Could you check a few things on this model? Use its own coordinates, in mm. A direction names the side the tool comes from. Coordinates: 2 decimals unless noted, no trailing zeros. Write each loop counter-clockwise with the first axis right and the second up, starting at its lowest first coordinate (ties: lowest second). Pieces come first, ordered by that corner, then holes. Notation, with made-up numbers: M -14.5,76.5 L 34.5,76.5 A26 cw 34.5,98.5 Z; hole C -29,23 d10. An arc over 180 degrees is marked long. Write item = value, one per line.
```python
from build123d import *

# Parameters (mm, degrees)
F1_DEPTH  = 25.4
F3_DEPTH  = 12.7
F5_DEPTH  = 12.7
F7_DEPTH  = 12.7
F9_DEPTH  = 12.7
F10_DEPTH = 12.7


with BuildPart() as f1:
    # F0 (on Top) → F1 (new body)
    with BuildSketch(Plane.XY):
        with BuildLine():
            ThreePointArc((0, 6.35), (1.8598719395, 1.8598719395), (6.35, 0))
            Line((6.35, 0), (69.85, 0))
            ThreePointArc((69.85, 0), (74.3401280605, 1.8598719395), (76.2, 6.35))
            Line((76.2, 6.35), (76.2, 12.7))
            Line((76.2, 12.7), (63.5, 12.7))
            Line((63.5, 12.7), (63.5, 25.4))
            Line((63.5, 25.4), (63.5, 38.1))
            Line((63.5, 38.1), (76.2, 38.1))
            Line((76.2, 38.1), (76.2, 44.45))
            ThreePointArc((76.2, 44.45), (74.3401280605, 48.9401280605), (69.85, 50.8))
            Line((69.85, 50.8), (6.35, 50.8))
            ThreePointArc((6.35, 50.8), (1.8598719395, 48.9401280605), (0, 44.45))
            Line((0, 44.45), (0, 38.1))
            Line((0, 38.1), (12.7, 38.1))
            Line((12.7, 38.1), (12.7, 25.4))
            Line((12.7, 25.4), (12.7, 12.7))
            Line((12.7, 12.7), (0, 12.7))
            Line((0, 12.7), (0, 6.35))
        make_face()
    extrude(amount=F1_DEPTH)

    # F2 (on face) → F3 (join)
    with BuildSketch(Plane(origin=(0, 0, 0), x_dir=(1, 0, 0), z_dir=(0, 0, -1))):
        Polygon((63.5, -12.7), (63.5, 0), (50.8120395243, 0), (50.8120395243, -50.8), (63.5, -50.8), (63.5, -38.1), align=None)
        Polygon((25.4, -50.8), (25.4, 0), (12.7, 0), (12.7, -12.7), (12.7, -38.1), (12.7, -50.8), align=None)
    extrude(amount=F3_DEPTH)

    # F4 (on face) → F5 (join)
    with BuildSketch(Plane.XY.offset(25.4)):
        Polygon((19.5285081863, 50.8), (38.1, 0), (53.2767996192, 50.8), align=None)
    extrude(amount=F5_DEPTH)

    # F6 (on face) → F7 (join)
    with BuildSketch(Plane.XY.offset(38.1)):
        Polygon((19.5285081863, 50.8), (28.8142540932, 25.4), (45.6883998096, 25.4), (53.2767996192, 50.8), align=None)
    extrude(amount=F7_DEPTH)

    # F10 (add): a face of the model
    f10_faces = [f1.faces().sort_by_distance(p)[0] for p in [
        (36.7798419244, 39.5111111111, 50.8),
    ]]


with BuildPart() as f9:
    # F8 (on face) → F9 (new body)
    with BuildSketch(Plane.XY.offset(50.8)):
        Polygon((45.6883998096, 25.4), (28.8142540932, 25.4), (37.9194319248, 0), align=None)
    extrude(amount=F9_DEPTH)


with BuildPart() as f1_1:
    add(f1.part)

    add(f9.part)  # F10 merges F9
    extrude(f10_faces, amount=F10_DEPTH)


solid = f1_1.part
```
Item 1: I'm going to push flat-ended pins straight in: P1, Ø4, axis at x = 30, y = 34.5, coming from the -Z side; P2, Ø4, axis at x = 36.5, z = 44, coming from the -Y side; P3, Ø19, axis at y = 28, z = 8, coming from the +X side. Where does each tip first touch, or does it pass through?
Numbers:
P1 = 0
P2 = 25.4
P3 = 63.5
Item 2: If I drill on line 1 along Y through (x, z) = (11, 8); line 2 along Z through (x, y) = (32, 12); line 3 along X through (y, z) = (46.5, -1), over which ranges is the centre line in solid material (lowest first)?
Numbers:
line_1 = 0 to 12.7, 38.1 to 50.8
line_2 = 0 to 25.4
line_3 = 12.7 to 25.4, 50.81 to 63.5
Item 3: Imagine slicing it at B-B (y = 17.5). Write out the boundary of the cut face in (x, z).
Numbers:
outline = M 12.7,-12.7 L 25.4,-12.7 L 25.4,0 L 50.81,0 L 50.81,-12.7 L 63.5,-12.7 L 63.5,25.4 L 43.33,25.4 L 43.33,38.1 L 31.7,38.1 L 31.7,25.4 L 12.7,25.4 Z; M 31.65,50.8 L 43.27,50.8 L 43.27,63.5 L 31.65,63.5 Z
Item 4: For faces 1 (the face through (6, 45, 0)), 2 (the face through (6, 38.1, 13)), 3 (the face through (25.4, 26, -6)), which set-ups out of +Z, -Z, +X, -X, +Y, -Y let a thin tool reach every point of the face, with its end or its side?
Numbers:
face_1 = -Z, -X, +Y, -Y
face_2 = +Z, -Z, -X
face_3 = -Z, +Y, -Y
Item 5: Imagine slicing it at A-A (x = 65.5). Write out the boundary of the cut face in (y, z).
Numbers:
outline = M 0,0 L 12.7,0 L 12.7,25.4 L 0,25.4 Z; M 38.1,0 L 50.8,0 L 50.8,25.4 L 38.1,25.4 Z
Item 6: If we mould it in two halves opening along Z, with no side actions, what happens to faces 4 (the face through (0, 41, 13)), 5 (the face through (37, 19, 38.1)), 6 (the face through (38, 26, 0)), 7 (the face through (37, 19, 50.8))? For each: pulls with the +Z half, pulls with the -Z half, needs draft (parallel to the pull), parting line crosses it, or undercut.
Numbers:
face_4 = needs draft
face_5 = undercut
face_6 = pulls with the -Z half
face_7 = undercut
Item 7: Imagine slicing it at D-D (y = 27). Write out the boundary of the cut face in (x, z).
Numbers:
outline = M 12.7,-12.7 L 25.4,-12.7 L 25.4,0 L 50.81,0 L 50.81,-12.7 L 63.5,-12.7 L 63.5,25.4 L 46.17,25.4 L 46.17,63.5 L 28.23,63.5 L 28.23,25.4 L 12.7,25.4 Z
Item 8: Imagine slicing it at C-C (z = 12). Write out the boundary of the cut face in (x, y).
Numbers:
outline = M 0,6.35 A6.35 ccw 6.35,0 L 69.85,0 A6.35 ccw 76.2,6.35 L 76.2,12.7 L 63.5,12.7 L 63.5,38.1 L 76.2,38.1 L 76.2,44.45 A6.35 ccw 69.85,50.8 L 6.35,50.8 A6.35 ccw 0,44.45 L 0,38.1 L 12.7,38.1 L 12.7,12.7 L 0,12.7 Z
